```python
from build123d import *

# Parameters (mm, degrees)
BOSS_EXTRUDE1_DEPTH = 4
CUT_EXTRUDE1_DEPTH  = 10


with BuildPart() as part:
    # Sketch1 → Boss-Extrude1 (new body)
    with BuildSketch(Plane(origin=(0, 0, 0), x_dir=(1, 0, 0), z_dir=(0, 1, 0))):
        Polygon((-10.4, 13.35), (-10.4, 11.35), (-14.4, 11.35), (-14.4, 7.35), (-10.4, 7.35), (-10.4, 3.35), (-14.4, 3.35), (-14.4, -0.65), (-10.4, -0.65), (-10.4, -4.65), (-14.4, -4.65), (-14.4, -8.65), (-10.4, -8.65), (-10.4, -12.65), (-14.4, -12.65), (-14.4, -16.65), (-10.4, -16.65), (-10.4, -20.65), (-14.4, -20.65), (-14.4, -24.65), (-10.4, -24.65), (-10.4, -28.65), (-14.4, -28.65), (-14.4, -32.65), (-10.4, -32.65), (-10.4, -36.65), (-14.4, -36.65), (-14.4, -40.65), (-10.4, -40.65), (-10.4, -44.65), (-14.4, -44.65), (-14.4, -48.65), (-10.4, -48.65), (-10.4, -52.65), (-14.4, -52.65), (-14.4, -56.65), (-10.4, -56.65), (-10.4, -60.65), (79.6, -60.65), (79.6, -56.65), (83.6, -56.65), (83.6, -52.65), (79.6, -52.65), (79.6, -40.65), (83.6, -40.65), (83.6, -36.65), (79.6, -36.65), (79.6, -24.65), (83.6, -24.65), (83.6, -20.65), (79.6, -20.65), (79.6, -8.65), (83.6, -8.65), (83.6, -4.65), (79.6, -4.65), (79.6, 7.35), (83.6, 7.35), (83.6, 11.35), (79.6, 11.35), (79.6, 13.35), align=None)
    extrude(amount=-BOSS_EXTRUDE1_DEPTH)

    # Sketch2 → Cut-Extrude1 (cut)
    with BuildSketch(Plane(origin=(0, 0, 0), x_dir=(1, 0, 0), z_dir=(0, 1, 0))):
        with BuildLine():
            Line((1.986692504, 9.35), (29.6, 9.35))
            ThreePointArc((29.6, 9.35), (31.014213562, 8.764213562), (31.6, 7.35))
            Line((31.6, 7.35), (31.6, -13.44487837))
            ThreePointArc((31.6, -13.44487837), (30.492669396, -15.23461057), (28.39685865, -15.042517532))
            Line((28.39685865, -15.042517532), (0.783551154, 5.752360838))
            ThreePointArc((0.783551154, 5.752360838), (0.089948145, 7.984319192), (1.986692504, 9.35))
        make_face()
        with BuildLine():
            ThreePointArc((-6.4, 2.14487837), (-5.292669396, 3.93461057), (-3.19685865, 3.742517532))
            Line((-3.19685865, 3.742517532), (24.416448846, -17.052360838))
            ThreePointArc((24.416448846, -17.052360838), (25.110051855, -19.284319192), (23.213307496, -20.65))
            Line((23.213307496, -20.65), (-4.4, -20.65))
            ThreePointArc((-4.4, -20.65), (-5.814213562, -20.064213562), (-6.4, -18.65))
            Line((-6.4, -18.65), (-6.4, 2.14487837))
        make_face()
        with BuildLine():
            Line((37.6, 7.35), (37.6, -13.44487837))
            ThreePointArc((37.6, -13.44487837), (38.707330604, -15.23461057), (40.80314135, -15.042517532))
            Line((40.80314135, -15.042517532), (68.416448846, 5.752360838))
            ThreePointArc((68.416448846, 5.752360838), (69.110051855, 7.984319192), (67.213307496, 9.35))
            Line((67.213307496, 9.35), (39.6, 9.35))
            ThreePointArc((39.6, 9.35), (38.185786438, 8.764213562), (37.6, 7.35))
        make_face()
        with BuildLine():
            ThreePointArc((75.6, -18.65), (75.014213562, -20.064213562), (73.6, -20.65))
            Line((73.6, -20.65), (45.986692504, -20.65))
            ThreePointArc((45.986692504, -20.65), (44.089948145, -19.284319192), (44.783551154, -17.052360838))
            Line((44.783551154, -17.052360838), (72.39685865, 3.742517532))
            ThreePointArc((72.39685865, 3.742517532), (74.492669396, 3.93461057), (75.6, 2.14487837))
            Line((75.6, 2.14487837), (75.6, -18.65))
        make_face()
        with BuildLine():
            ThreePointArc((75.6, -49.44487837), (74.492669396, -51.23461057), (72.39685865, -51.042517532))
            Line((72.39685865, -51.042517532), (44.783551154, -30.247639162))
            ThreePointArc((44.783551154, -30.247639162), (44.089948145, -28.015680808), (45.986692504, -26.65))
            Line((45.986692504, -26.65), (73.6, -26.65))
            ThreePointArc((73.6, -26.65), (75.014213562, -27.235786438), (75.6, -28.65))
            Line((75.6, -28.65), (75.6, -49.44487837))
        make_face()
        with BuildLine():
            Line((67.213307496, -56.65), (39.6, -56.65))
            ThreePointArc((39.6, -56.65), (38.185786438, -56.064213562), (37.6, -54.65))
            Line((37.6, -54.65), (37.6, -33.85512163))
            ThreePointArc((37.6, -33.85512163), (38.707330604, -32.06538943), (40.80314135, -32.257482468))
            Line((40.80314135, -32.257482468), (68.416448846, -53.052360838))
            ThreePointArc((68.416448846, -53.052360838), (69.110051855, -55.284319192), (67.213307496, -56.65))
        make_face()
        with BuildLine():
            Line((31.6, -54.65), (31.6, -33.85512163))
            ThreePointArc((31.6, -33.85512163), (30.492669396, -32.06538943), (28.39685865, -32.257482468))
            Line((28.39685865, -32.257482468), (0.783551154, -53.052360838))
            ThreePointArc((0.783551154, -53.052360838), (0.089948145, -55.284319192), (1.986692504, -56.65))
            Line((1.986692504, -56.65), (29.6, -56.65))
            ThreePointArc((29.6, -56.65), (31.014213562, -56.064213562), (31.6, -54.65))
        make_face()
        with BuildLine():
            ThreePointArc((-6.4, -28.65), (-5.814213562, -27.235786438), (-4.4, -26.65))
            Line((-4.4, -26.65), (23.213307496, -26.65))
            ThreePointArc((23.213307496, -26.65), (25.110051855, -28.015680808), (24.416448846, -30.247639162))
            Line((24.416448846, -30.247639162), (-3.19685865, -51.042517532))
            ThreePointArc((-3.19685865, -51.042517532), (-5.292669396, -51.23461057), (-6.4, -49.44487837))
            Line((-6.4, -49.44487837), (-6.4, -28.65))
        make_face()
    extrude(amount=-CUT_EXTRUDE1_DEPTH, mode=Mode.SUBTRACT)


solid = part.part
```
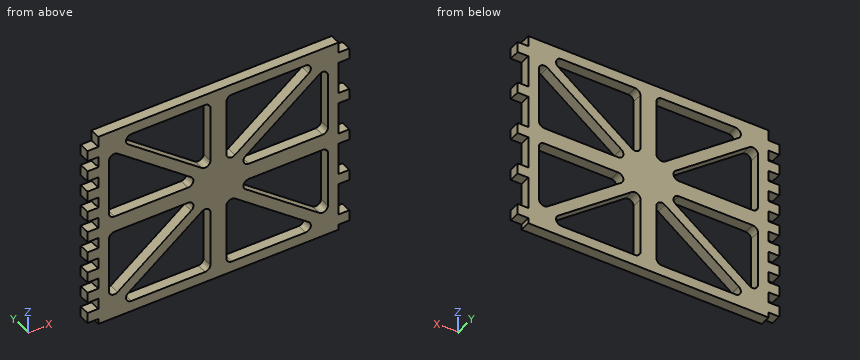
Geometry check sheet. Reference: the model listing, model coordinates, mm. Give positions to 0.01 mm unless a question says otherwise; leave off trailing zeros. Order: outer loops, then holes, each group sorted by start corner. A loop starts at its lowest first (then second) coordinate and runs counter-clockwise, first axis right, second up. Notation, with made-up numbers: (5, -21) - (61, -21) arc R18 ccw to (61, -1) - close; hole circle Ø1 at (-37, 36.25). An arc over 180 degrees is marked (long way). Write item = value, one per line. Start each with the question number.
1) Gauge pin test, flat ends, axial feed: pin 1 Ø2 at (x, y) = (-12.5, -2.5) entering from -Z; pin 2 Ø1.2 at (x, y) = (81, -2) entering from +Z; pin 3 Ø2 at (y, z) = (-1.5, 49) entering from +X. Record the tip position at first contact, or that the pin passes through.
2) Section check A-A (x = 3). Enter the section's corners in (y, z).
3) Section check B-B (z = 46.5). Enter the section's corners in (x, y).
4) Scan lines: L1, parallel to X at y = -2.6, z = 18.5; L2, parallel to X at y = -1.1, z = 54.5; L3, parallel to Z at x = 62, y = -1.15. Record each from-to range of solid material in increasing order.
5) Section check C-C (y = -2.9). Count the separate pieces of the cut face and the enclosed holes in it, then the cut area to 3 significant figures.
6) Section check D-D (x = 27). Enter the section's corners in (y, z), then the cut area to 3 significant figures.
Geometry check:
q1.pin_1 = -11.35
q1.pin_2 = 56.65
q1.pin_3 = 79.6
q2.outline = (-4, -13.35) - (0, -13.35) - (0, -9.35) - (-4, -9.35) - close; (-4, -4.08) - (0, -4.08) - (0, 0.92) - (-4, 0.92) - close; (-4, 20.65) - (0, 20.65) - (0, 26.65) - (-4, 26.65) - close; (-4, 46.38) - (0, 46.38) - (0, 51.38) - (-4, 51.38) - close; (-4, 56.65) - (0, 56.65) - (0, 60.65) - (-4, 60.65) - close
q3.outline = (-14.4, -4) - (-6.4, -4) - (-6.4, 0) - (-14.4, 0) - close; (2.84, -4) - (9.48, -4) - (9.48, 0) - (2.84, 0) - close; (31.6, -4) - (37.6, -4) - (37.6, 0) - (31.6, 0) - close; (59.72, -4) - (66.36, -4) - (66.36, 0) - (59.72, 0) - close; (75.6, -4) - (79.6, -4) - (79.6, 0) - (75.6, 0) - close
q4.L1 = -10.4 to -6.4, 25.21 to 43.99, 75.6 to 79.6
q4.L2 = -14.4 to -0.01, 31.6 to 37.6, 69.21 to 83.6
q4.L3 = -13.35 to -9.35, -0.92 to 4.09, 20.65 to 26.65, 43.21 to 48.22, 56.65 to 60.65
q5.separate_pieces = 1
q5.enclosed_holes = 8
q5.area = 3,160 mm2
q6.outline = (-4, -13.35) - (0, -13.35) - (0, -9.35) - (-4, -9.35) - close; (-4, 13.99) - (0, 13.99) - (0, 33.31) - (-4, 33.31) - close; (-4, 56.65) - (0, 56.65) - (0, 60.65) - (-4, 60.65) - close
q6.area = 109 mm2
